```python
from build123d import *

# Parameters (mm, degrees)
F1_DEPTH = 200


with BuildPart() as f1:
    # F0 (on Front) → F1 (new body)
    with BuildSketch(Plane.XZ):
        with BuildLine():
            Line((6.35, -10.9985226281), (0, -7.3323484187))
            Line((0, -7.3323484187), (-6.35, -10.9985226281))
            Line((-6.35, -10.9985226281), (-6.35, -73.65))
            ThreePointArc((-6.35, -73.65), (0, -80), (6.35, -73.65))
            Line((6.35, -73.65), (6.35, -10.9985226281))
        make_face()
        Polygon((-6.35, -10.9985226281), (0, -7.3323484187), (-3.175, -5.499261314), (-6.35, -3.6661742094), align=None)
        Polygon((3.175, -5.499261314), (0, -7.3323484187), (6.35, -10.9985226281), (6.35, -3.6661742094), align=None)
        with BuildLine():
            Line((-6.35, 10.9985226281), (0, 7.3323484187))
            Line((0, 7.3323484187), (6.35, 10.9985226281))
            Line((6.35, 10.9985226281), (6.35, 73.65))
            ThreePointArc((6.35, 73.65), (0, 80), (-6.35, 73.65))
            Line((-6.35, 73.65), (-6.35, 10.9985226281))
        make_face()
        Polygon((6.35, 10.9985226281), (0, 7.3323484187), (3.175, 5.499261314), (6.35, 3.6661742094), align=None)
        Polygon((-3.175, 5.499261314), (0, 7.3323484187), (-6.35, 10.9985226281), (-6.35, 3.6661742094), align=None)
        with BuildLine():
            Line((-6.35, -10.9985226281), (-6.35, -3.6661742094))
            Line((-6.35, -3.6661742094), (-12.7, 0))
            Line((-12.7, 0), (-66.9577709887, -31.325738686))
            ThreePointArc((-66.9577709887, -31.325738686), (-69.2820323028, -40), (-60.6077709887, -42.324261314))
            Line((-60.6077709887, -42.324261314), (-6.35, -10.9985226281))
        make_face()
        Polygon((-12.7, 0), (-6.35, -3.6661742094), (-6.35, 0), (-6.35, 3.6661742094), align=None)
        Polygon((6.35, 0), (6.35, -3.6661742094), (12.7, 0), (6.35, 3.6661742094), align=None)
        with BuildLine():
            Line((12.7, 0), (6.35, -3.6661742094))
            Line((6.35, -3.6661742094), (6.35, -10.9985226281))
            Line((6.35, -10.9985226281), (60.6077709887, -42.324261314))
            ThreePointArc((60.6077709887, -42.324261314), (69.2820323028, -40), (66.9577709887, -31.325738686))
            Line((66.9577709887, -31.325738686), (12.7, 0))
        make_face()
        with BuildLine():
            Line((-12.7, 0), (-6.35, 3.6661742094))
            Line((-6.35, 3.6661742094), (-6.35, 10.9985226281))
            Line((-6.35, 10.9985226281), (-60.6077709887, 42.324261314))
            ThreePointArc((-60.6077709887, 42.324261314), (-69.2820323028, 40), (-66.9577709887, 31.325738686))
            Line((-66.9577709887, 31.325738686), (-12.7, 0))
        make_face()
        with BuildLine():
            Line((6.35, 10.9985226281), (6.35, 3.6661742094))
            Line((6.35, 3.6661742094), (12.7, 0))
            Line((12.7, 0), (66.9577709887, 31.325738686))
            ThreePointArc((66.9577709887, 31.325738686), (69.2820323028, 40), (60.6077709887, 42.324261314))
            Line((60.6077709887, 42.324261314), (6.35, 10.9985226281))
        make_face()
    extrude(amount=F1_DEPTH)


solid = f1.part
```
The model under review builds one solid part; all positions refer to its coordinate system, in mm. A direction names the side the tool comes from. Give positions to 0.01 mm unless a question says otherwise; leave off trailing zeros. Loops run counter-clockwise (first coordinate to the right, second up) from the corner with the lowest first, then second, coordinate; pieces in that order, holes last. Notation, with made-up numbers: (15.5, 13.5) - (38.5, 13.5) arc R22 ccw to (38.5, 36.5) - close; hole circle Ø1 at (-7.75, 65.5). An arc over 180 degrees is marked (long way). Answer as a JSON object with one key per item and string values.
Q1. Mouldability with a two-part tool opening along Z and no side actions: class faces 6 (the cylindrical face through (0, -99, 80)), 7 (the flat face through (6.35, -99, 42)), 8 (the flat face through (-39.449, -98.6, -15.444)) as +Z half, -Z half, draft (parallel to the pull), parting line (faces both ways), or undercut.
Worked out:
{"face 6": "+Z half", "face 7": "draft", "face 8": "undercut"}
Q2. Add section B-B on z = -17. State the section outline as (x, y) points, plus the area to 3 significant figures.
Worked out:
{"outline": "(-42.14, -200) - (-16.74, -200) - (-16.74, 0) - (-42.14, 0) - close; (-6.35, -200) - (6.35, -200) - (6.35, 0) - (-6.35, 0) - close; (16.74, -200) - (42.14, -200) - (42.14, 0) - (16.74, 0) - close", "area": "12,700 mm^2"}
Q3. Insertion check: pin 1 (19 mm diameter, centred on y = -75, z = 57.5, fed in from -X); pin 2 (5 mm diameter, centred on y = -108, z = -22, fed in from +X); pin 3 (2 mm diameter, centred on x = 10, y = -168.5, fed in from +Z); pin 4 (5 mm diameter, centred on y = -33, z = -37, fed in from -X). Each pin has a flat end and moves straight along its axis. Give the tip position at first contact, or say it passes through.
Worked out:
{"pin 1": "stops at x = -6.35", "pin 2": "stops at x = 55.14", "pin 3": "stops at z = 13.68", "pin 4": "stops at x = -70.13"}
Q4. Add section C-C on x = -55. State the section outline as (y, z) points, plus the area to 3 significant figures.
Worked out:
{"outline": "(-200, -39.09) - (0, -39.09) - (0, -24.42) - (-200, -24.42) - close; (-200, 24.42) - (0, 24.42) - (0, 39.09) - (-200, 39.09) - close", "area": "5,870 mm^2"}
Q5. To check wall thickness, follow line 1 along X through (y, z) = (-118.5, -36.5); line 2 along X through (y, z) = (-157.5, 29.5); line 3 along Z through (x, y) = (0, -155.5). State the ranges of each line that lie inside material, in increasing order.
Worked out:
{"line 1": "x = -70.12 to -50.52, -6.35 to 6.35, 50.52 to 70.12", "line 2": "x = -63.8 to -38.4, -6.35 to 6.35, 38.4 to 63.8", "line 3": "z = -80 to -7.33, 7.33 to 80"}
Q6. Add section D-D on z = -39. State the section outline as (x, y) points, plus the area to 3 significant figures.
Worked out:
{"outline": "(-69.75, -200) - (-54.85, -200) - (-54.85, 0) - (-69.75, 0) - close; (-6.35, -200) - (6.35, -200) - (6.35, 0) - (-6.35, 0) - close; (54.85, -200) - (69.75, -200) - (69.75, 0) - (54.85, 0) - close", "area": "8,500 mm^2"}
Q7. For faces 1 (the flat face through (33.86, -98.6, 26.88)), 2 (the flat face through (-33.86, -98.6, -26.88)), 3 (the flat face through (-40.209, -98.6, 15.882)), 4 (the flat face through (-6.35, -99, 0)), 5 (the flat face through (40.209, -98.6, -15.882)), list the 3-axis set-ups (+Z, -Z, +X, -X, +Y, -Y) from which the entire face can be reached by the end or side of a thin tool; tool diameter is ignored.
Worked out:
{"face 1": "+Z, +Y, -Y", "face 2": "-Z, +Y, -Y", "face 3": "-X, +Y, -Y", "face 4": "+Y, -Y", "face 5": "+X, +Y, -Y"}
Q8. Add section A-A on y = -171.5. State the section outline as (x, z) points (3 decimals), plus the area to 3 significant figures.
Worked out:
{"outline": "(-66.958, -31.326) arc R6.35 ccw to (-60.608, -42.324) - (-6.35, -10.999) - (-6.35, -73.65) arc R6.35 ccw to (6.35, -73.65) - (6.35, -10.999) - (60.608, -42.324) arc R6.35 ccw to (66.958, -31.326) - (12.7, 0) - (66.958, 31.326) arc R6.35 ccw to (60.608, 42.324) - (6.35, 10.999) - (6.35, 73.65) arc R6.35 ccw to (-6.35, 73.65) - (-6.35, 10.999) - (-60.608, 42.324) arc R6.35 ccw to (-66.958, 31.326) - (-12.7, 0) - close; hole (-6.35, -3.666) - (0, -7.332) - (6.35, -3.666) - (6.35, 3.666) - (0, 7.332) - (-6.35, 3.666) - close", "area": "5,430 mm^2"}
